from build123d import *

# Parameters (mm, degrees)
SKETCH1_W                      = 50
SKETCH1_H                      = 30
BASE_FLANGE1_DEPTH             = 1
EDGE_FLANGE1_STRIP_W           = 8
EDGE_FLANGE1_STRIP_H           = 1
EDGE_FLANGE1_STRIP_CUT_DEPTH   = 30
EDGE_FLANGE1_STRIP_2_W         = 8
EDGE_FLANGE1_STRIP_2_H         = 1
EDGE_FLANGE1_STRIP_CUT_2_DEPTH = 30
EDGE_FLANGE1_DEPTH             = 30
EDGE_FLANGE1_BEND_DEPTH        = 30
EDGE_FLANGE2_STRIP_W           = 5.4732
EDGE_FLANGE2_STRIP_H           = 1
EDGE_FLANGE2_STRIP_CUT_DEPTH   = 30
EDGE_FLANGE2_STRIP_2_W         = 5.4732
EDGE_FLANGE2_STRIP_2_H         = 1
EDGE_FLANGE2_STRIP_CUT_2_DEPTH = 30
EDGE_FLANGE2_DEPTH             = 30
EDGE_FLANGE2_BEND_DEPTH        = 30
EDGE_FLANGE3_DEPTH             = 44
EDGE_FLANGE4_DEPTH             = 6
EDGE_FLANGE4_START             = 1
EDGE_FLANGE4_PROFILE_R         = 2.5
EDGE_FLANGE4_FLAT_DEPTH        = 1
CUT_EXTRUDE1_DEPTH             = 60.36539396
CUT_EXTRUDE1_DEPTH_BACK        = 60.36539396
SKETCH38_R                     = 2.5
FILLET1_R                      = 6


# Sheet-metal steps are written as plain solids
with BuildPart() as part:
    # Sketch1 → Base-Flange1 (new body)
    with BuildSketch(Plane(origin=(0, 0, 0), x_dir=(1, 0, 0), z_dir=(0, 1, 0))):
        Rectangle(SKETCH1_W, SKETCH1_H)
    extrude(amount=-BASE_FLANGE1_DEPTH)

    # Edge-Flange1 strip (across the edge) → Edge-Flange1 strip cut (cut)
    with BuildSketch(Plane(origin=(25, 0, 15), x_dir=(-1, 0, 0), z_dir=(0, 0, -1))):
        with Locations((-1, -0.5)):
            Rectangle(EDGE_FLANGE1_STRIP_W, EDGE_FLANGE1_STRIP_H)
    extrude(amount=EDGE_FLANGE1_STRIP_CUT_DEPTH, mode=Mode.SUBTRACT)

    # Edge-Flange1 strip 2 (across the edge) → Edge-Flange1 strip cut 2 (cut)
    with BuildSketch(Plane(origin=(-25, 0, -15), x_dir=(1, 0, 0), z_dir=(0, 0, 1))):
        with Locations((-1, -0.5)):
            Rectangle(EDGE_FLANGE1_STRIP_2_W, EDGE_FLANGE1_STRIP_2_H)
    extrude(amount=EDGE_FLANGE1_STRIP_CUT_2_DEPTH, mode=Mode.SUBTRACT)

    # Edge-Flange1 section (across the edge) → Edge-Flange1 (add)
    with BuildSketch(Plane(origin=(25, 0, 15), x_dir=(-1, 0, 0), z_dir=(0, 0, -1))):
        with BuildLine():
            Line((0, 2), (0, 19))
            Line((0, 19), (1, 19))
            Line((1, 19), (1, 2))
            ThreePointArc((1, 2), (1.585786438, 0.585786438), (3, 0))
            Line((3, 0), (3, -1))
            ThreePointArc((3, -1), (0.878679656, -0.121320344), (0, 2))
        make_face()
    extrude(amount=EDGE_FLANGE1_DEPTH)

    # Edge-Flange1 section 2 (across the edge) → Edge-Flange1 bend (add)
    with BuildSketch(Plane(origin=(-25, 0, -15), x_dir=(1, 0, 0), z_dir=(0, 0, 1))):
        with BuildLine():
            Line((0, 2), (0, 19))
            Line((0, 19), (1, 19))
            Line((1, 19), (1, 2))
            ThreePointArc((1, 2), (1.585786438, 0.585786438), (3, 0))
            Line((3, 0), (3, -1))
            ThreePointArc((3, -1), (0.878679656, -0.121320344), (0, 2))
        make_face()
    extrude(amount=EDGE_FLANGE1_BEND_DEPTH)

    # Edge-Flange2 strip (across the edge) → Edge-Flange2 strip cut (cut)
    with BuildSketch(Plane(origin=(25, 19, -15), x_dir=(0, -1, 0), z_dir=(0, 0, 1))):
        with Locations((-2, -0.5)):
            Rectangle(EDGE_FLANGE2_STRIP_W, EDGE_FLANGE2_STRIP_H)
    extrude(amount=EDGE_FLANGE2_STRIP_CUT_DEPTH, mode=Mode.SUBTRACT)

    # Edge-Flange2 strip 2 (across the edge) → Edge-Flange2 strip cut 2 (cut)
    with BuildSketch(Plane(origin=(-25, 19, 15), x_dir=(0, -1, 0), z_dir=(0, 0, -1))):
        with Locations((-2, -0.5)):
            Rectangle(EDGE_FLANGE2_STRIP_2_W, EDGE_FLANGE2_STRIP_2_H)
    extrude(amount=EDGE_FLANGE2_STRIP_CUT_2_DEPTH, mode=Mode.SUBTRACT)

    # Edge-Flange2 section (across the edge) → Edge-Flange2 (add)
    with BuildSketch(Plane(origin=(25, 19, -15), x_dir=(0, -1, 0), z_dir=(0, 0, 1))):
        with BuildLine():
            Line((-1, 0.7366), (-1, 16.5))
            Line((-1, 16.5), (0, 16.5))
            Line((0, 16.5), (0, 0.7366))
            ThreePointArc((0, 0.7366), (0.215745145, 0.215745145), (0.7366, 0))
            Line((0.7366, 0), (0.7366, -1))
            ThreePointArc((0.7366, -1), (-0.491361636, -0.491361636), (-1, 0.7366))
        make_face()
    extrude(amount=EDGE_FLANGE2_DEPTH)

    # Edge-Flange2 section 2 (across the edge) → Edge-Flange2 bend (add)
    with BuildSketch(Plane(origin=(-25, 19, 15), x_dir=(0, -1, 0), z_dir=(0, 0, -1))):
        with BuildLine():
            Line((-1, 0.7366), (-1, 16.5))
            Line((-1, 16.5), (0, 16.5))
            Line((0, 16.5), (0, 0.7366))
            ThreePointArc((0, 0.7366), (0.215745145, 0.215745145), (0.7366, 0))
            Line((0.7366, 0), (0.7366, -1))
            ThreePointArc((0.7366, -1), (-0.491361636, -0.491361636), (-1, 0.7366))
        make_face()
    extrude(amount=EDGE_FLANGE2_BEND_DEPTH)

    # Edge-Flange3 section (across the edge) → Edge-Flange3 (add)
    with BuildSketch(Plane(origin=(22, -1, 16), x_dir=(0, 0, -1), z_dir=(-1, 0, 0))):
        with BuildLine():
            Line((-1, 1), (-1, 14))
            Line((-1, 14), (0, 14))
            Line((0, 14), (0, 1))
            ThreePointArc((0, 1), (0.292893219, 0.292893219), (1, 0))
            Line((1, 0), (1, -1))
            ThreePointArc((1, -1), (-0.414213562, -0.414213562), (-1, 1))
        make_face()
    extrude(amount=EDGE_FLANGE3_DEPTH)

    # Edge-Flange4 bend section (across the edge) → Edge-Flange4 (add)
    with BuildSketch(Plane(origin=(-22.7366, -9, 17), x_dir=(1, 0, 0), z_dir=(0, -1, 0))):
        with BuildLine():
            Line((-1, 0.7366), (0, 0.7366))
            ThreePointArc((0, 0.7366), (0.215745145, 0.215745145), (0.7366, 0))
            Line((0.7366, 0), (0.7366, -1))
            ThreePointArc((0.7366, -1), (-0.491361636, -0.491361636), (-1, 0.7366))
        make_face()
    edge_flange4 = extrude(amount=EDGE_FLANGE4_DEPTH)

    # Edge-Flange4 profile (on flange) → Edge-Flange4 flat (add)
    with BuildSketch(Plane(origin=(-22.7366, 0, 17), x_dir=(0, -1, 0), z_dir=(-1, 0, 0)).offset(EDGE_FLANGE4_START)):
        with BuildLine():
            Line((9, 14), (9, 0.7366))
            Line((9, 0.7366), (15, 0.7366))
            Line((15, 0.7366), (15, 4))
            Line((15, 4), (24, 4))
            ThreePointArc((24, 4), (29, 9), (24, 14))
            Line((24, 14), (9, 14))
        make_face()
        with Locations((24, 9)):
            Circle(EDGE_FLANGE4_PROFILE_R, mode=Mode.SUBTRACT)
    edge_flange4_flat = extrude(amount=-EDGE_FLANGE4_FLAT_DEPTH)

    # Mirror1: Edge-Flange4, Edge-Flange4 flat across plane
    add(edge_flange4.mirror(Plane(origin=(0, 0, 0), x_dir=(0, 0, 1), z_dir=(1, 0, 0))))
    add(edge_flange4_flat.mirror(Plane(origin=(0, 0, 0), x_dir=(0, 0, 1), z_dir=(1, 0, 0))))

    # Sketch38 → Cut-Extrude1 (cut, two sides: drawn at the far end of the back side and taken through both)
    with BuildSketch(Plane(origin=(0, 0, 0), x_dir=(1, 0, 0), z_dir=(0, 1, 0)).offset(-CUT_EXTRUDE1_DEPTH_BACK)):
        with Locations(Location((-35.5, 9, 0), (0, 0, 270))):
            Circle(SKETCH38_R)
        with Locations(Location((-35.5, -9, 0), (0, 0, 270))):
            Circle(SKETCH38_R)
        with BuildLine():
            Line((-9, -8), (9, -8))
            ThreePointArc((9, -8), (17, 0), (9, 8))
            Line((9, 8), (-9, 8))
            ThreePointArc((-9, 8), (-17, 0), (-9, -8))
        make_face()
        with Locations(Location((35.5, 9, 0), (0, 0, 270))):
            Circle(SKETCH38_R)
        with Locations(Location((35.5, -9, 0), (0, 0, 270))):
            Circle(SKETCH38_R)
    extrude(amount=CUT_EXTRUDE1_DEPTH + CUT_EXTRUDE1_DEPTH_BACK, mode=Mode.SUBTRACT)

    # Fillet1
    fillet1_edges = [part.edges().sort_by_distance(p)[0] for p in [
        (41.5, 19.5, -15),
        (41.5, 19.5, 15),
        (-41.5, 19.5, 15),
        (-41.5, 19.5, -15),
    ]]
    fillet(fillet1_edges, radius=FILLET1_R)


solid = part.part
Geometry check sheet. Reference: the model listing, model coordinates, mm. A direction names the side the tool comes from. Coordinates: 2 decimals unless noted, no trailing zeros. Order: outer loops, then holes, each group sorted by start corner. A loop starts at its lowest first (then second) coordinate and runs counter-clockwise, first axis right, second up. Notation, with made-up numbers: (5, -15) -> (59, -15) arc R18 ccw to (59, 14) -> close; hole circle Ø10 at (-22.5, -28.75). An arc over 180 degrees is marked (long way). Use a Markdown table: item, result. Add a question column.
1. Material ranges on L1, parallel to Z at x = -35.5, y = 19.45; L2, parallel to X at y = 11, z = -7.5; L3, parallel to Z at x = -23, y = -24, recorded low to high.
2. Mould release check, pull along Z, two halves, no side actions. Record for faces 6 (the face through (-33.39, 19.49, 10.34)), 7 (the face through (0.31, -0.57, 16.4)), 8 (the face through (-23.43, 0.6, -0.21)): pulls with the +Z half, pulls with the -Z half, needs draft (parallel to the pull), parting line crosses it, or undercut.
3. Cross-section at D-D (z = 3). Enter the section's corners in (x, y), and give its area (3 significant figures).
4. Set-up check for faces 1 (the face through (-24, 10, 0)), 2 (the face through (25, 10, 0)), 3 (the face through (-25, 10, 0)), 4 (the face through (23.737, -17, 26)), 5 (the face through (22.737, -17, 26)): record each of +Z, -Z, +X, -X, +Y, -Y from which the full face is reachable in a straight line by a thin tool's end or side.
5. Cross-section at B-B (y = 6). Enter the section's corners in (x, z), and give its area (3 significant figures).
6. Cross-section at A-A (z = 26). Enter the section's corners in (x, y).
7. Go/stop test with flat-tipped pins: pin 1 Ø6 at (y, z) = (-19, 19.5) entering from -X; pin 2 Ø12.5 at (x, z) = (-36.5, -6.5) entering from -Y; pin 3 Ø2 at (x, y) = (10, -12.5) entering from -Z. Record where each tip stops, or that it passes through.
8. Cross-section at C-C (x = -6.5). Enter the section's corners in (y, z), and give its area (3 significant figures).
Filled sheet:
| question | item | result |
|---|---|---|
| 1 | L1 | -15 to -11.5, -6.5 to 6.5, 11.5 to 15 |
| 1 | L2 | -25 to -24, 24 to 25 |
| 1 | L3 | 21 to 23.5, 28.5 to 31 |
| 2 | face 6 | undercut |
| 2 | face 7 | pulls with the +Z half |
| 2 | face 8 | needs draft |
| 3 | outline | (-41.5, 19) -> (-25.74, 19) arc R0.74 cw to (-25, 18.26) -> (-25, 2) arc R3 ccw to (-22, -1) -> (-16.42, -1) -> (-16.42, 0) -> (-22, 0) arc R2 cw to (-24, 2) -> (-24, 18.26) arc R1.74 ccw to (-25.74, 20) -> (-41.5, 20) -> close; (16.42, -1) -> (22, -1) arc R3 ccw to (25, 2) -> (25, 18.26) arc R0.74 cw to (25.74, 19) -> (41.5, 19) -> (41.5, 20) -> (25.74, 20) arc R1.74 ccw to (24, 18.26) -> (24, 2) arc R2 cw to (22, 0) -> (16.42, 0) -> close |
| 3 | area | 87.0 mm2 |
| 4 | face 1 | +Z, -Z, +Y |
| 4 | face 2 | +Z, -Z, +X, -Y |
| 4 | face 3 | +Z, -Z, -X, -Y |
| 4 | face 4 | +Z, -Z, +X, +Y, -Y |
| 4 | face 5 | +Z, +Y, -Y |
| 5 | outline | (-25, -15) -> (-24, -15) -> (-24, 15) -> (-25, 15) -> close; (24, -15) -> (25, -15) -> (25, 15) -> (24, 15) -> close |
| 5 | area | 60.0 mm2 |
| 6 | outline | (-23.74, -29) -> (-22.74, -29) -> (-22.74, -26.5) -> (-23.74, -26.5) -> close; (-23.74, -21.5) -> (-22.74, -21.5) -> (-22.74, -9) -> (-23.74, -9) -> close; (22.74, -29) -> (23.74, -29) -> (23.74, -26.5) -> (22.74, -26.5) -> close; (22.74, -21.5) -> (23.74, -21.5) -> (23.74, -9) -> (22.74, -9) -> close |
| 7 | pin 1 | x = -23.74 |
| 7 | pin 2 | y = 19 |
| 7 | pin 3 | z = 16 |
| 8 | outline | (-15, 16) -> (-2, 16) arc R1 cw to (-1, 15) -> (-1, 8) -> (0, 8) -> (0, 15) arc R2 ccw to (-2, 17) -> (-15, 17) -> close; (-1, -15) -> (0, -15) -> (0, -8) -> (-1, -8) -> close |
| 8 | area | 29.4 mm2 |
